Work out the finished part from the listing and answer in its coordinate system (mm). A direction names the side the tool comes from. Give positions to 0.01 mm unless a question says otherwise; leave off trailing zeros. Write each loop counter-clockwise with the first axis right and the second up, starting at its lowest first coordinate (ties: lowest second). Pieces come first, ordered by that corner, then holes. Notation, with made-up numbers: (13, 64.25) - (27, 64.25) arc R34 cw to (27, 101.25) - close; hole circle Ø9 at (-22.5, -19.5). An arc over 180 degrees is marked (long way). Write each question's results on one line, items separated by ' | '. Start each with the question number.
from build123d import *

# Parameters (mm, degrees)
SKETCH1_W                 = 10
SKETCH1_H                 = 14
EXTRUDE1_DEPTH            = 56.7
SKETCH2_W                 = 10
SKETCH2_H                 = 18.498
EXTRUDE2_DEPTH            = 3
M3X0_5_TAPPED_HOLE1_D     = 2.5
M3X0_5_TAPPED_HOLE1_DEPTH = 7.5
M3X0_5_TAPPED_HOLE1_TIP   = 0.220408726
M3X0_5_TAPPED_HOLE2_D     = 2.5
M3X0_5_TAPPED_HOLE2_DEPTH = 7.5
M3X0_5_TAPPED_HOLE2_TIP   = 0.220408726


with BuildPart() as part:
    # Sketch1 → Extrude1 (new body)
    with BuildSketch(Plane(origin=(0, 0, 0), x_dir=(1, 0, 0), z_dir=(0, 1, 0))):
        Rectangle(SKETCH1_W, SKETCH1_H)
    extrude(amount=-EXTRUDE1_DEPTH)

    # Sketch2 → Extrude2 (add)
    with BuildSketch(Plane.XY.offset(7)):
        with Locations((0, -13.249)):
            Rectangle(SKETCH2_W, SKETCH2_H)
    extrude(amount=EXTRUDE2_DEPTH)

    # M3x0.5 Tapped Hole1
    with Locations(Plane(origin=(0, -36.2, -7), x_dir=(-1, 0, 0), z_dir=(0, 0, -1))):
        with Locations((0, 0), (0, -6.4), (0, -12.8)):
            Hole(M3X0_5_TAPPED_HOLE1_D / 2, depth=M3X0_5_TAPPED_HOLE1_DEPTH)
            with Locations((0, 0, -(M3X0_5_TAPPED_HOLE1_DEPTH + M3X0_5_TAPPED_HOLE1_TIP / 2))):  # 160° drill point
                Cone(0, M3X0_5_TAPPED_HOLE1_D / 2, M3X0_5_TAPPED_HOLE1_TIP, mode=Mode.SUBTRACT)

    # M3x0.5 Tapped Hole2
    with Locations(Plane.XY.offset(7)):
        with Locations((2, -39.4), (-2, -45.81)):
            Hole(M3X0_5_TAPPED_HOLE2_D / 2, depth=M3X0_5_TAPPED_HOLE2_DEPTH)
            with Locations((0, 0, -(M3X0_5_TAPPED_HOLE2_DEPTH + M3X0_5_TAPPED_HOLE2_TIP / 2))):  # 160° drill point
                Cone(0, M3X0_5_TAPPED_HOLE2_D / 2, M3X0_5_TAPPED_HOLE2_TIP, mode=Mode.SUBTRACT)


solid = part.part
Q1. The mould has two halves that part along X. Classify faces 1 (the conical face through (-0.036, -42.669, 0.707)), 2 (the flat face through (0, -28, -7)), 3 (the flat face through (-5, -28, 0)): pulls with the +X half, pulls with the -X half, needs draft (parallel to the pull), parting line crosses it, or undercut.
Q2. A tool of negligible diameter and unlimited length cuts with its end or side. For faces 4 (the cylindrical face through (-0.16, -41.36, -3.2)), 5 (the cylindrical face through (2.27, -40.62, 3.2)), 6 (the flat face through (0, -22.498, 8)), from which of +Z, -Z, +X, -X, +Y, -Y can it reach the whole face along a straight path? Write none if from no direction.
Q3. A cutting plane is placed at B-B, the plane x = 4.25. Write down the section's boundary in (y, z), and give its area (3 significant figures).
Q4. Given pin 1 (2.5 mm diameter, centred on x = 2.5, z = 8.5, fed in from -Y); pin 2 (5 mm diameter, centred on x = -0.5, y = -37, fed in from +Z); pin 3 (1.5 mm diameter, centred on x = 0, y = -36.2, fed in from -Z), each flat-ended and moving along its own axis, determine where each tip first touches the part or whether it passes through.
Q5. A cutting plane is placed at D-D, the plane y = -53. Write down the section's boundary in (x, z).
Q6. A cutting plane is placed at C-C, the plane z = 2.5. Write down the section's boundary in (x, y).
Q7. A cutting plane is placed at A-A, the plane z = -1.5. Write down the section's boundary in (x, y), and give its area (3 significant figures).
Q8. Consider L1, parallel to Y at x = 0, z = -1.25; L2, parallel to Y at x = 0.75, z = -6; L3, parallel to X at y = -45.81, z = 4.5. Determine where each line is inside the solid, lowest interval first.
Result:
1) face 1: undercut | face 2: needs draft | face 3: pulls with the -X half
2) face 4: -Z | face 5: +Z | face 6: +Z, +X, -X, -Y
3) outline: (-56.7, -7) - (0, -7) - (0, 7) - (-4, 7) - (-4, 10) - (-22.5, 10) - (-22.5, 7) - (-56.7, 7) - close | area: 849 mm2
4) pin 1: stops at y = -22.5 | pin 2: stops at z = 7 | pin 3: stops at z = 0.59
5) outline: (-5, -7) - (5, -7) - (5, 7) - (-5, 7) - close
6) outline: (-5, -56.7) - (5, -56.7) - (5, 0) - (-5, 0) - close; hole circle Ø2.5 at (-2, -45.81); hole circle Ø2.5 at (2, -39.4)
7) outline: (-5, -56.7) - (5, -56.7) - (5, 0) - (-5, 0) - close; hole circle Ø2.5 at (0, -49); hole circle Ø2.5 at (0, -42.6); hole circle Ø2.5 at (0, -36.2) | area: 552 mm2
8) L1: y = -56.7 to -50.25, -47.75 to -43.85, -41.35 to -37.45, -34.95 to 0 | L2: y = -56.7 to -50, -48 to -43.6, -41.6 to -37.2, -35.2 to 0 | L3: x = -5 to -3.25, -0.75 to 5
